```python
from build123d import *

# Parameters (mm, degrees)
SKETCH1_R             = 1.6
BOSS_EXTRUDE1_DEPTH   = 8
M6X1_0_TAPPED_HOLE1_D = 5
CIRPATTERN4_COUNT     = 4


with BuildPart() as part:
    # Sketch1 → Boss-Extrude1 (new body)
    with BuildSketch(Plane.XY):
        with BuildLine():
            Line((-29.326822194, 5), (-20.106608804, 5))
            ThreePointArc((-20.106608804, 5), (-19.399502023, 4.707106781), (-19.106608804, 4))
            Line((-19.106608804, 4), (-19.106608804, -4))
            ThreePointArc((-19.106608804, -4), (-19.399502023, -4.707106781), (-20.106608804, -5))
            Line((-20.106608804, -5), (-29.326822194, -5))
            ThreePointArc((-29.326822194, -5), (-21.03642674, -21.03642674), (-5, -29.326822194))
            Line((-5, -29.326822194), (-5, -20.106608804))
            ThreePointArc((-5, -20.106608804), (-4.707106781, -19.399502023), (-4, -19.106608804))
            Line((-4, -19.106608804), (4, -19.106608804))
            ThreePointArc((4, -19.106608804), (4.707106781, -19.399502023), (5, -20.106608804))
            Line((5, -20.106608804), (5, -29.326822194))
            ThreePointArc((5, -29.326822194), (21.03642674, -21.03642674), (29.326822194, -5))
            Line((29.326822194, -5), (20.106608804, -5))
            ThreePointArc((20.106608804, -5), (19.399502023, -4.707106781), (19.106608804, -4))
            Line((19.106608804, -4), (19.106608804, 4))
            ThreePointArc((19.106608804, 4), (19.399502023, 4.707106781), (20.106608804, 5))
            Line((20.106608804, 5), (29.326822194, 5))
            ThreePointArc((29.326822194, 5), (21.03642674, 21.03642674), (5, 29.326822194))
            Line((5, 29.326822194), (5, 20.106608804))
            ThreePointArc((5, 20.106608804), (4.707106781, 19.399502023), (4, 19.106608804))
            Line((4, 19.106608804), (-4, 19.106608804))
            ThreePointArc((-4, 19.106608804), (-4.707106781, 19.399502023), (-5, 20.106608804))
            Line((-5, 20.106608804), (-5, 29.326822194))
            ThreePointArc((-5, 29.326822194), (-21.03642674, 21.03642674), (-29.326822194, 5))
        make_face()
        with Locations((13.965358928, 13.965358928)):
            Circle(SKETCH1_R, mode=Mode.SUBTRACT)
        with Locations((13.965358928, -13.965358928)):
            Circle(SKETCH1_R, mode=Mode.SUBTRACT)
        with Locations((-13.965358928, -13.965358928)):
            Circle(SKETCH1_R, mode=Mode.SUBTRACT)
        with Locations((-13.965358928, 13.965358928)):
            Circle(SKETCH1_R, mode=Mode.SUBTRACT)
    extrude(amount=BOSS_EXTRUDE1_DEPTH)

    # M6x1.0 Tapped Hole1 (through all)
    with Locations(Plane.XY.offset(8)):
        with Locations((0, 0)):
            Hole(M6X1_0_TAPPED_HOLE1_D / 2)

    # Sketch10 → M3x0.5 Tapped Hole2 (revolve, cut)
    with BuildSketch(Plane(origin=(-21.03642674, -21.03642674, 3), x_dir=(0.707106781186559, -0.707106781186536, 0), z_dir=(0, 0, 1))):
        Polygon((0, 0), (0, 7), (1.25, 6.248924226), (1.25, 0), align=None)
    m3x0_5_tapped_hole2 = revolve(axis=Axis((-25.526554801, -25.526554801, 3), (0.707106781186536, 0.707106781186559, 0)), mode=Mode.SUBTRACT)

    # CirPattern4: M3x0.5 Tapped Hole2 ×4 about axis
    cirpattern4_axis = Axis((0, 0, 8), (0, 0, -1))
    for i in range(1, CIRPATTERN4_COUNT):
        add(m3x0_5_tapped_hole2.rotate(cirpattern4_axis, i * 360 / CIRPATTERN4_COUNT), mode=Mode.SUBTRACT)


solid = part.part
```
Here's how the part is built. I have some questions about the finished solid (model axes, mm). A direction names the side the tool comes from. Give positions to 0.01 mm unless a question says otherwise; leave off trailing zeros. Write each loop counter-clockwise with the first axis right and the second up, starting at its lowest first coordinate (ties: lowest second). Pieces come first, ordered by that corner, then holes. Notation, with made-up numbers: M 4,50.25 L 34,50.25 A12 ccw 34,73.25 Z; hole C 57.25,57 d9. An arc over 180 degrees is marked long. Put each result on its own line as item: value. Start each with the question number.
Item 1: If we section it at A-A, the plane x = 0: Write out the boundary of the cut face in (y, z), then the cut area to 3 significant figures.
Item 2: If we section it at D-D, the plane x = 10: Write out the boundary of the cut face in (y, z), then the cut area to 3 significant figures.
Item 3: Thinking about a two-plate mould opening in Z: for faces 1 (the flat face through (0, -6, 8)), 2 (the flat face through (-5, -25, 4)), 3 (the cylindrical face through (18.207, -19.51, 2.155)), which applies, +Z half, -Z half, draft (parallel to the pull), parting line (faces both ways), or undercut?
Item 4: Will these pins go through, and if not, where does the flat tip stop? pin 1 (2 mm diameter, centred on y = 0, z = 1, fed in from +X); pin 2 (2 mm diameter, centred on x = -12, z = 3.5, fed in from +Y); pin 3 (2.5 mm diameter, centred on x = -1, z = 4.5, fed in from -Y); pin 4 (6 mm diameter, centred on x = 0, y = 0, fed in from +Z).
Item 5: I need wall thicknesses on L1, parallel to Y at x = -17, z = 2.5; L2, parallel to X at y = 17, z = 3.75; L3, parallel to X at y = -13, z = 6.5. Which ranges of each line are inside material? Lowest first, please. Write a range as from..to.
Item 6: On a 3-axis mill with a long thin cutter (end or side, diameter ignored), from which of +Z, -Z, +X, -X, +Y, -Y can I reach the whole of each face in a straight line? I mean faces 4 (the flat face through (5, 25, 4)), 5 (the flat face through (25, 5, 4)), 6 (the flat face through (-25, 5, 4)), 7 (the conical face through (16.07, -16.29, 2.85)). Say none if no direction works.
Item 7: If we section it at C-C, the plane z = 6.5: Count the separate pieces of the cut face and the enclosed holes in it, then the cut area to 3 significant figures.
Values:
1. outline: M -19.11,0 L -2.5,0 L -2.5,8 L -19.11,8 Z; M 2.5,0 L 19.11,0 L 19.11,8 L 2.5,8 Z
1. area: 266 mm²
2. outline: M -28.02,0 L 28.02,0 L 28.02,8 L -28.02,8 Z
2. area: 448 mm²
3. face 1: +Z half
3. face 2: draft
3. face 3: undercut
4. pin 1: x = 19.11
4. pin 2: y = 27.64
4. pin 3: y = -19.11
4. pin 4: z = 8
5. L1: -24.41..-18.62, -15.94..15.94, 18.62..24.41
5. L2: -24.41..-18.41, -16.03..16.03, 18.41..24.41
5. L3: -26.76..-15.24, -12.69..12.69, 15.24..26.76
6. face 4: +Z, -Z, +Y
6. face 5: +Z, -Z, +X
6. face 6: +Z, -Z, -X
6. face 7: none
7. separate pieces: 1
7. enclosed holes: 5
7. area: 2,310 mm²
